Work out the finished part from the listing and answer in its coordinate system (mm). Face numbers are marked on the shaded views. A direction names the side the tool comes from. Coordinates: 2 decimals unless noted, no trailing zeros. Order: outer loops, then holes, each group sorted by start corner. A loop starts at its lowest first (then second) coordinate and runs counter-clockwise, first axis right, second up. Notation, with made-up numbers: M 72,68.5 L 78,68.5 A5 cw 78,75.5 Z; hole C 58.25,4 d8. An arc over 180 degrees is marked long. Answer in a Markdown table with one row per item. Add a question column.
Item 1: The mould has two halves that part along X. Classify the marked faces 1, 2 and 3: released by +X, released by -X, zero draft, split by the parting line, or undercut.
Item 2: The part is cut by section A-A (x = 20.5). Write down the section's boundary in (y, z), then the cut area to 3 significant figures.
Item 3: The part is cut by section C-C (x = 14.5). Write down the section's boundary in (y, z).
Item 4: The part is cut by section B-B (y = 0). Write down the section's boundary in (x, z), then the cut area to 3 significant figures.
Item 5: Consider line 1 (X direction, y = 18, z = 2.5); line 2 (Y direction, x = 25, z = 2.5); line 3 (Y direction, x = 7, z = 1.5). Determine where each line is inside the solid, lowest interval first. Write a range as from..to.
Item 6: Flat-ended cylindrical pins translate along their axes: pin 1 Ø3 at (x, z) = (18.5, 6.5) entering from -Y; pin 2 Ø0.5 at (x, y) = (25.5, 15) entering from +Z; pin 3 Ø4 at (y, z) = (25, 11.5) entering from +X; pin 4 Ø4 at (x, y) = (14.5, -2.5) entering from -Z. Find the tip coordinate at first contact, or state that the pin passes through.
Item 7: Which of the six approach directions +Z, -Z, +X, -X, +Y, -Y give full straight-line access (tool end or side, diameter ignored) to the marked faces 4, 5, 6 and 7?
Item 8: The part is cut by section D-D (z = 12). State how many separate pieces and enclosed holes the cut face has, then the cut area to 3 significant figures.
from build123d import *

# Parameters (mm, degrees)
F2_ANGLE = 180
F3_ANGLE = -180
F1_W     = 1.832515
F1_H     = 4.050821
F1_W_2   = 1.832514
F4_DEPTH = 0.25


with BuildPart() as f2:
    # F0 (on Top) → F2 (revolve)
    with BuildSketch(Plane.XY):
        with BuildLine():
            ThreePointArc((30, 11.4), (29.56066, 12.46066), (28.5, 12.9))
            Line((28.5, 12.9), (23.800393, 12.9))
            Line((23.800393, 12.9), (23.800393, 11.4))
            Line((23.800393, 11.4), (19.800393, 11.4))
            Line((19.800393, 11.4), (19.800393, 12.9))
            Line((19.800393, 12.9), (5.840044, 12.9))
            Line((5.840044, 12.9), (5.840044, 11.4))
            Line((5.840044, 11.4), (1.840044, 11.4))
            Line((1.840044, 11.4), (1.840044, 12.9))
            Line((1.840044, 12.9), (0, 12.9))
            ThreePointArc((0, 12.9), (-1.06066, 12.46066), (-1.5, 11.4))
            Line((-1.5, 11.4), (-1.5, 6.9))
            Line((-1.5, 6.9), (0, 6.9))
            Line((0, 6.9), (0, 8.8))
            Line((0, 8.8), (12.214104, 8.2))
            Line((12.214104, 8.2), (30, 8.2))
            Line((30, 8.2), (30, 11.4))
        make_face()
    revolve(axis=Axis((15, 0, 0), (1, 0, 0)), revolution_arc=F2_ANGLE)



with BuildPart() as f3:
    # F0 (on Top) → F3 (revolve)
    with BuildSketch(Plane.XY):
        with BuildLine():
            Line((19.800393, 17.768246), (23.800393, 17.768246))
            Line((23.800393, 17.768246), (23.800393, 16.268246))
            Line((23.800393, 16.268246), (28.5, 16.268246))
            ThreePointArc((28.5, 16.268246), (29.56066, 16.707586), (30, 17.768246))
            Line((30, 17.768246), (30, 20.968246))
            Line((30, 20.968246), (12.214104, 20.968246))
            Line((12.214104, 20.968246), (0, 20.368246))
            Line((0, 20.368246), (0, 22.268246))
            Line((0, 22.268246), (-1.5, 22.268246))
            Line((-1.5, 22.268246), (-1.5, 17.768246))
            ThreePointArc((-1.5, 17.768246), (-1.06066, 16.707586), (0, 16.268246))
            Line((0, 16.268246), (1.840044, 16.268246))
            Line((1.840044, 16.268246), (1.840044, 17.768246))
            Line((1.840044, 17.768246), (5.840044, 17.768246))
            Line((5.840044, 17.768246), (5.840044, 16.268246))
            Line((5.840044, 16.268246), (19.800393, 16.268246))
            Line((19.800393, 16.268246), (19.800393, 17.768246))
        make_face()
    revolve(axis=Axis((15, 29.168246, 0), (1, 0, 0)), revolution_arc=F3_ANGLE)


with BuildPart() as f2_1:
    add(f2.part)

    add(f3.part)  # F4 merges F3
    # F1 (on Top) → F4 (join)
    with BuildSketch(Plane.XY):
        with Locations((26.144934, 14.680172)):
            Rectangle(F1_W, F1_H)
        with Locations((9.618169, 14.680172)):
            Rectangle(F1_W_2, F1_H)
    extrude(amount=F4_DEPTH)


solid = f2_1.part
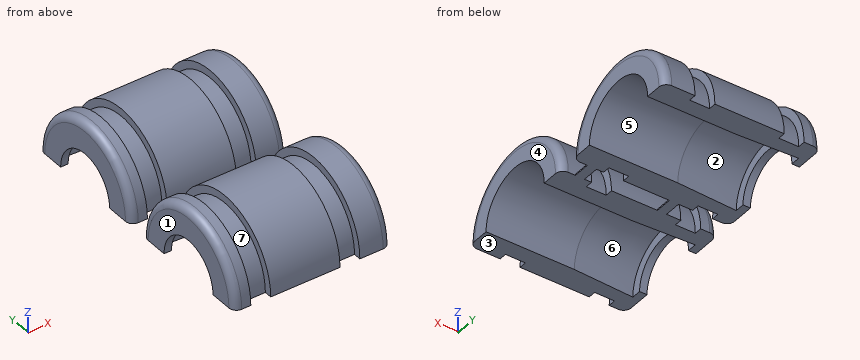
Reply:
| question | item | result |
|---|---|---|
| 1 | face 1 | released by -X |
| 1 | face 2 | undercut |
| 1 | face 3 | zero draft |
| 2 | outline | M -11.4,0 L -8.2,0 A8.2 cw 8.2,0 L 11.4,0 A11.4 ccw Z; M 17.77,0 L 20.97,0 A8.2 cw 37.37,0 L 40.57,0 A11.4 ccw Z |
| 2 | area | 197 mm2 |
| 3 | outline | M -12.9,0 L -8.2,0 A8.2 cw 8.2,0 L 12.9,0 A12.9 ccw Z; M 16.27,0 L 20.97,0 A8.2 cw 37.37,0 L 42.07,0 A12.9 ccw Z |
| 4 | outline | M -1.5,6.9 L 0,6.9 L 0,8.8 L 12.21,8.2 L 30,8.2 L 30,11.4 A1.5 ccw 28.5,12.9 L 23.8,12.9 L 23.8,11.4 L 19.8,11.4 L 19.8,12.9 L 5.84,12.9 L 5.84,11.4 L 1.84,11.4 L 1.84,12.9 L 0,12.9 A1.5 ccw -1.5,11.4 Z |
| 4 | area | 133 mm2 |
| 5 | line 1 | x = -1.5..1.84, 5.84..19.8, 23.8..30 |
| 5 | line 2 | y = -12.66..-7.81, 7.81..12.66, 16.51..21.36, 36.98..41.82 |
| 5 | line 3 | y = -12.81..-8.32, 8.32..12.81, 16.36..20.85, 37.49..41.98 |
| 6 | pin 1 | stops at y = -11.89 |
| 6 | pin 2 | stops at z = 0.25 |
| 6 | pin 3 | stops at x = 30 |
| 6 | pin 4 | stops at z = 6.85 |
| 7 | face 4 | +Z, -Z, +X, +Y, -Y |
| 7 | face 5 | -Z, +X |
| 7 | face 6 | -Z |
| 7 | face 7 | +Z |
| 8 | separate pieces | 6 |
| 8 | enclosed holes | 0 |
| 8 | area | 431 mm2 |
